Geometry: see drawing. Coordinates: mm, zero at the bounding-box minimum. A direction names the side the tool comes from. Coordinates: 2 decimals unless noted, no trailing zeros. Order: outer loops, then holes, each group sorted by start corner. A loop starts at its lowest first (then second) coordinate and runs counter-clockwise, first axis right, second up. Notation, with made-up numbers: M -33,5.25 L -6,5.25 A26 cw -6,25.25 Z; hole C 8,-15 d5. An arc over 180 degrees is marked long. Answer in a Markdown table with one row per item.
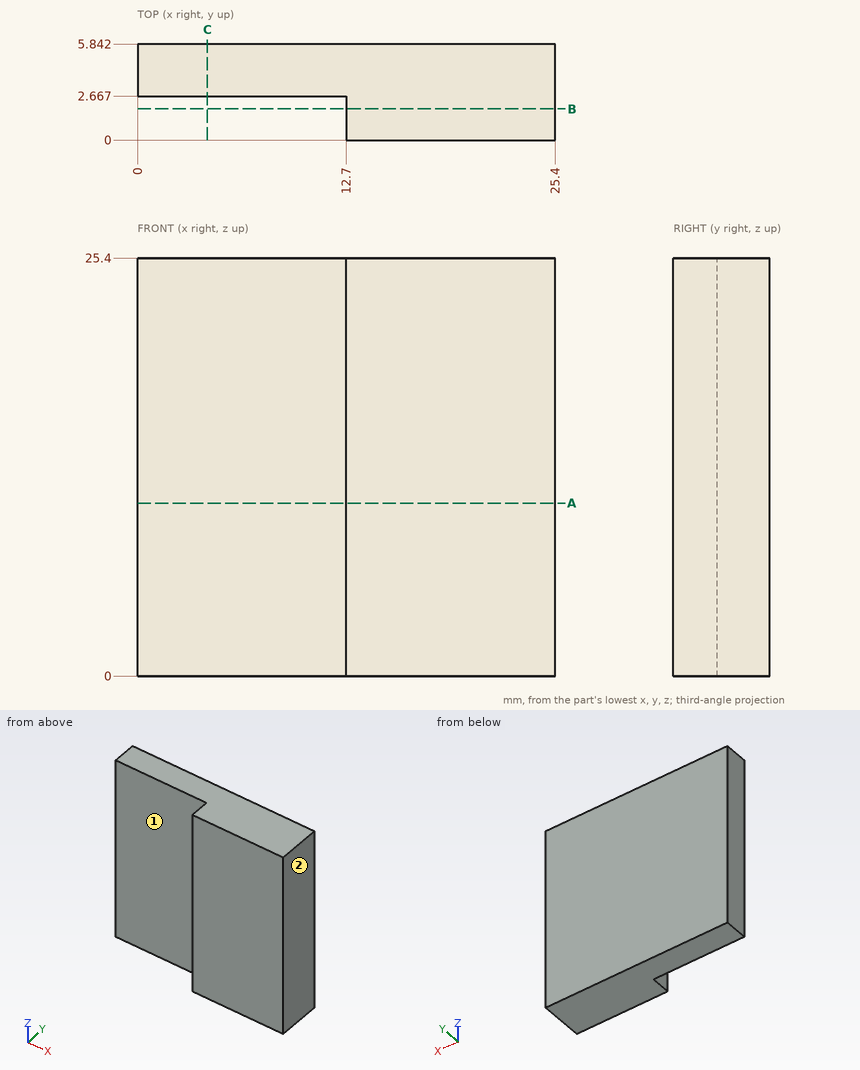
1) Cut plane A-A, the plane z = 10.5. Output: boundary loops of the cut face in (x, y), and give its area (3 significant figures).
Resolved:
| item | result |
|---|---|
| outline | M 0,2.67 L 12.7,2.67 L 12.7,0 L 25.4,0 L 25.4,5.84 L 0,5.84 Z |
| area | 115 mm2 |
2) Reachability of the marked faces 1 and 2 from +Z, -Z, +X, -X, +Y, -Y: full face, straight path, thin tool, end or side. Return the list, or none.
Resolved:
| item | result |
|---|---|
| face 1 | +Z, -Z, -X, -Y |
| face 2 | +Z, -Z, +X, +Y, -Y |
3) Cut plane C-C, the plane x = 4.25. Output: boundary loops of the cut face in (y, z).
Resolved:
| item | result |
|---|---|
| outline | M 2.67,0 L 5.84,0 L 5.84,25.4 L 2.67,25.4 Z |
4) Cut plane B-B, the plane y = 1.9. Output: boundary loops of the cut face in (x, z).
Resolved:
| item | result |
|---|---|
| outline | M 12.7,0 L 25.4,0 L 25.4,25.4 L 12.7,25.4 Z |
5) Material intervals for probe 1 along X at (y, z) = (2.25, 3); probe 2 along Y at (x, z) = (8.75, 23.75), sorted ascending.
Resolved:
| item | result |
|---|---|
| probe 1 | x = 12.7 to 25.4 |
| probe 2 | y = 2.67 to 5.84 |
6) Contact query for a flat-ended pin moving along its axis: pin 1 (4 mm diameter, centred on x = 9, z = 14, fed in from -Y). Output: stop coordinate, or through.
Resolved:
| item | result |
|---|---|
| pin 1 | stops at y = 2.67 |
